Geometry check sheet. Reference: drawing and pictorial views, mm from the part's lowest x, y, z. A direction names the side the tool comes from. Give positions to 0.01 mm unless a question says otherwise; leave off trailing zeros. Loops run counter-clockwise (first coordinate to the right, second up) from the corner with the lowest first, then second, coordinate; pieces in that order, holes last. Notation, with made-up numbers: (42.5, -39.5) - (84.5, -39.5) arc R21 ccw to (84.5, -17.5) - close; hole circle Ø3 at (21, 55.5). An arc over 180 degrees is marked (long way). Answer in a Markdown table with one row per item. Add a question column.
(1) Set-up check for the marked faces 5 and 6: record each of +Z, -Z, +X, -X, +Y, -Y from which the full face is reachable in a straight line by a thin tool's end or side.
(2) Thickness scan on L1, parallel to Y at x = 4.25, z = 3.9 (3 decimals); L2, parallel to Z at x = 6.75, y = 4.5; L3, parallel to Y at x = 3.75, z = 73. Record the ranges inside material, lowest first.
(3) Draft check along Z on the marked faces 1, 2, 3 and 4. Enter one of: released by +Z, released by -Z, zero draft, split by the parting line, or undercut.
(4) Sectioned sample at A-A on y = 5.25. Enter the section's corners in (x, z), then the cut area to 3 significant figures.
(5) Sectioned sample at B-B on z = 48.5. Enter the section's corners in (x, y).
(6) Go/stop test with flat-tipped pins: P1, Ø2.5, axis at x = 4, z = 38, coming from the +Y side; P2, Ø2.5, axis at x = 6, z = 50, coming from the -Y side; P3, Ø2, axis at x = 4.25, y = 7.325, coming from the -Z side. Record where each tip stops, or that it passes through.
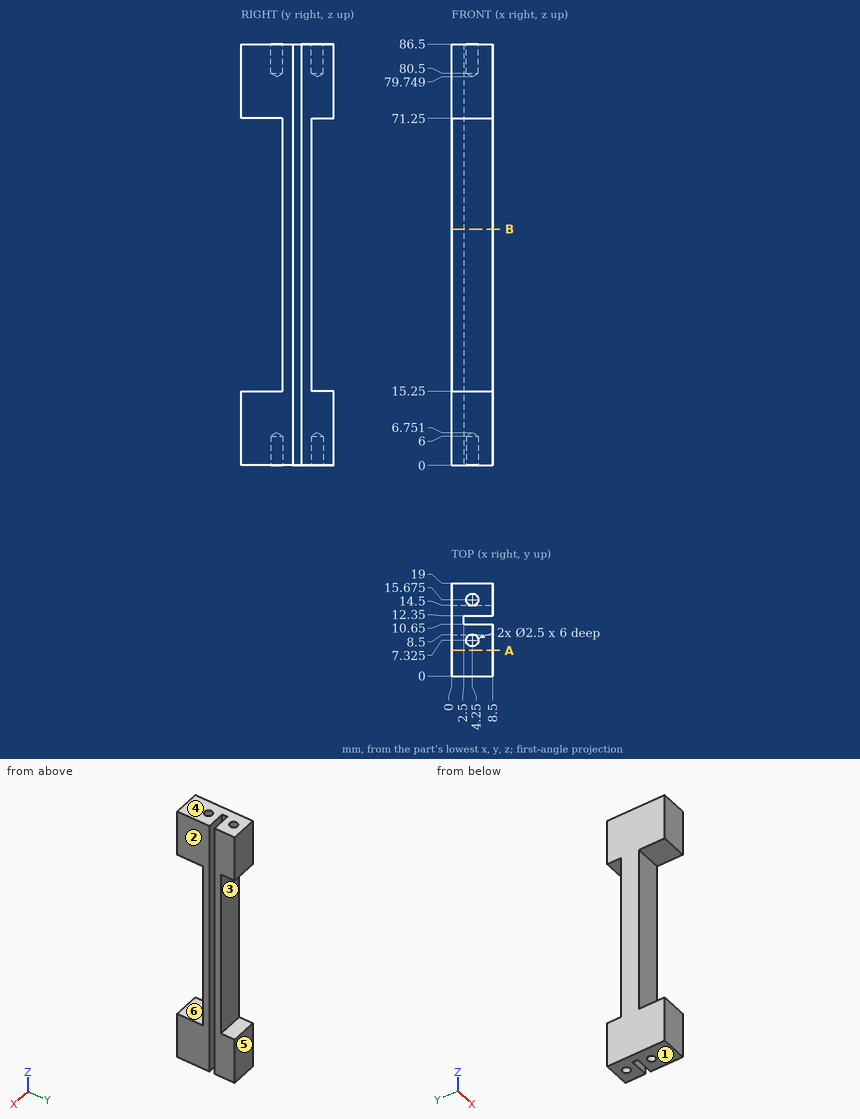
Reply:
| question | item | result |
|---|---|---|
| 1 | face 5 | +Z, -Z, +X, -X, +Y |
| 1 | face 6 | +X, -X, -Y |
| 2 | L1 | 0 to 6.075, 8.575 to 10.65, 12.35 to 14.425, 16.925 to 19 |
| 2 | L2 | 0 to 15.25, 71.25 to 86.5 |
| 2 | L3 | 0 to 10.65, 12.35 to 19 |
| 3 | face 1 | released by -Z |
| 3 | face 2 | zero draft |
| 3 | face 3 | undercut |
| 3 | face 4 | released by +Z |
| 4 | outline | (0, 0) - (8.5, 0) - (8.5, 15.25) - (0, 15.25) - close; (0, 71.25) - (8.5, 71.25) - (8.5, 86.5) - (0, 86.5) - close |
| 4 | area | 259 mm^2 |
| 5 | outline | (0, 8.5) - (8.5, 8.5) - (8.5, 10.65) - (2.5, 10.65) - (2.5, 12.35) - (8.5, 12.35) - (8.5, 14.5) - (0, 14.5) - close |
| 6 | P1 | y = 14.5 |
| 6 | P2 | y = 8.5 |
| 6 | P3 | z = 6.15 |
